The model under review builds one solid part; all positions refer to its coordinate system, in mm. A direction names the side the tool comes from. Round coordinates to 2 decimals unless told otherwise and drop trailing zeros. Write each loop counter-clockwise with the first axis right and the second up, starting at its lowest first coordinate (ties: lowest second). Pieces come first, ordered by that corner, then holes.
Item 1: Add section A-A (x = 139.5). Give the boundary of the cut face in (y, z), plus the area to 3 significant figures.
Item 2: Draft analysis for pull direction Z (two halves, no side actions). For faces 1 (the face through (103, 0, 1)), 2 (the face through (103, 0, 79)), 3 (the face through (103, 0, 0)), 4 (the face through (103, -12.681, 39)), state which applies: +Z half, -Z half, draft (parallel to the pull), parting line (faces both ways), or undercut.
Item 3: Add section B-B (z = 72). Give the boundary of the cut face in (x, y).
Item 4: To check wall thickness, follow L1, parallel to Z at x = 14.5, y = 9.25; L2, parallel to Y at x = 122, z = 71. State the ranges of each line that lie inside material, in increasing order.
Item 5: Add section C-C (y = 5.75). Give the boundary of the cut face in (x, z).
Item 6: Clearance check with a flat-ended pin moving along its axis: pin 1 Ø0.5 at (y, z) = (12, 46) entering from +X. State where the tip first meets the part, or that it passes through.
Item 7: Add section D-D (x = 103). Give the boundary of the cut face in (y, z).
Item 8: Machinability: for faces 5 (the face through (0, -11.4, 40.2)), 6 (the face through (103, 11.25, 41)), which of the approach directions +Z, -Z, +X, -X, +Y, -Y give a long, thin tool a straight path to every point of the face, cutting with its end or side? Answer none if there is none.
```python
from build123d import *

# Parameters (mm, degrees)
SKETCH_W        = 25
SKETCH_H        = 80
PAD_DEPTH       = 208
SKETCH001_W     = 22.5
SKETCH001_H     = 78
POCKET_DEPTH    = 1000
SKETCH002_W     = 58
SKETCH002_H     = 17
POCKET001_DEPTH = 26


with BuildPart() as part:
    # Sketch → Pad (new body)
    with BuildSketch(Plane.YZ):
        with Locations((-0.181115, 40)):
            Rectangle(SKETCH_W, SKETCH_H)
    extrude(amount=PAD_DEPTH)

    # Sketch001 (on Face5 of Pad) → Pocket (cut)
    with BuildSketch(Plane(origin=(0, 0, 0), x_dir=(0, 1, 0), z_dir=(-1, 0, 0))):
        with Locations((0, -40)):
            Rectangle(SKETCH001_W, SKETCH001_H)
    extrude(amount=-POCKET_DEPTH, mode=Mode.SUBTRACT)

    # Sketch002 (on Face2 of Pocket) → Pocket001 (cut)
    with BuildSketch(Plane(origin=(0, -12.681115, 0), x_dir=(0, 0, -1), z_dir=(0, -1, 0))):
        with Locations((-36, 16.5)):
            Rectangle(SKETCH002_W, SKETCH002_H)
        with Locations((-35.802797, 41.499222)):
            Rectangle(SKETCH002_W, SKETCH002_H)
        with Locations((-35.605594, 66.498444)):
            Rectangle(SKETCH002_W, SKETCH002_H)
        with Locations((-35.408391, 91.497667)):
            Rectangle(SKETCH002_W, SKETCH002_H)
        with Locations((-35.211188, 116.496889)):
            Rectangle(SKETCH002_W, SKETCH002_H)
        with Locations((-35.013985, 141.496111)):
            Rectangle(SKETCH002_W, SKETCH002_H)
        with Locations((-34.816782, 166.495333)):
            Rectangle(SKETCH002_W, SKETCH002_H)
        with Locations((-34.619579, 191.494555)):
            Rectangle(SKETCH002_W, SKETCH002_H)
        with Locations((-34.422376, 216.493778)):
            Rectangle(SKETCH002_W, SKETCH002_H)
        with Locations((-34.225173, 241.493)):
            Rectangle(SKETCH002_W, SKETCH002_H)
    extrude(amount=-POCKET001_DEPTH, mode=Mode.SUBTRACT)


solid = part.part
```
Numbers:
1. outline: (-12.68, 0) - (12.32, 0) - (12.32, 6.01) - (11.25, 6.01) - (11.25, 1) - (-11.25, 1) - (-11.25, 6.01) - (-12.68, 6.01) - close; (-12.68, 64.01) - (-11.25, 64.01) - (-11.25, 79) - (11.25, 79) - (11.25, 64.01) - (12.32, 64.01) - (12.32, 80) - (-12.68, 80) - close
1. area: 100 mm2
2. face 1: undercut
2. face 2: undercut
2. face 3: -Z half
2. face 4: draft
3. outline: (0, -12.68) - (208, -12.68) - (208, -11.25) - (0, -11.25) - close; (0, 11.25) - (208, 11.25) - (208, 12.32) - (0, 12.32) - close
4. L1: z = 0 to 1, 79 to 80
4. L2: y = -12.68 to -11.25, 11.25 to 12.32
5. outline: (0, 0) - (208, 0) - (208, 1) - (0, 1) - close; (0, 79) - (208, 79) - (208, 80) - (0, 80) - close
6. pin 1: stops at x = 207.99
7. outline: (-12.68, 0) - (12.32, 0) - (12.32, 80) - (-12.68, 80) - close; hole (-11.25, 1) - (11.25, 1) - (11.25, 79) - (-11.25, 79) - close
8. face 5: +Z, -Z, -X, +Y, -Y
8. face 6: +X, -X
